```python
from build123d import *

# Parameters (mm, degrees)
SKETCH1_W                      = 70
SKETCH1_H                      = 310
BASE_FLANGE1_DEPTH             = 0.81
EDGE_FLANGE1_STRIP_W           = 4.7132
EDGE_FLANGE1_STRIP_H           = 0.81
EDGE_FLANGE1_STRIP_CUT_DEPTH   = 310
EDGE_FLANGE1_DEPTH             = 310
EDGE_FLANGE2_STRIP_W           = 4.7132
EDGE_FLANGE2_STRIP_H           = 0.81
EDGE_FLANGE2_STRIP_CUT_DEPTH   = 310
EDGE_FLANGE2_DEPTH             = 310
EDGE_FLANGE3_STRIP_W           = 4.7132
EDGE_FLANGE3_STRIP_H           = 0.81
EDGE_FLANGE3_STRIP_CUT_DEPTH   = 68.4534
EDGE_FLANGE3_STRIP_2_W         = 4.7132
EDGE_FLANGE3_STRIP_2_H         = 0.81
EDGE_FLANGE3_STRIP_CUT_2_DEPTH = 68.4534
EDGE_FLANGE3_DEPTH             = 68.4534
EDGE_FLANGE3_BEND_DEPTH        = 68.4534
CUT_EXTRUDE2_REACH             = 325.201
SKETCH18_R                     = 2.5
SKETCH18_R_2                   = 1.5
CUT_EXTRUDE1_REACH             = 325.201
SKETCH17_R                     = 17.5
SKETCH17_R_2                   = 2.5
SKETCH17_R_3                   = 6


# Sheet-metal steps are written as plain solids
with BuildPart() as part:
    # Sketch1 → Base-Flange1 (new body)
    with BuildSketch(Plane.XY):
        with Locations((35, 155)):
            Rectangle(SKETCH1_W, SKETCH1_H)
    extrude(amount=-BASE_FLANGE1_DEPTH)

    # Edge-Flange1 strip (across the edge) → Edge-Flange1 strip cut (cut)
    with BuildSketch(Plane(origin=(0, 0, -0.81), x_dir=(1, 0, 0), z_dir=(0, 1, 0))):
        with Locations((-0.81, -0.405)):
            Rectangle(EDGE_FLANGE1_STRIP_W, EDGE_FLANGE1_STRIP_H)
    extrude(amount=EDGE_FLANGE1_STRIP_CUT_DEPTH, mode=Mode.SUBTRACT)

    # Edge-Flange1 section (across the edge) → Edge-Flange1 (add)
    with BuildSketch(Plane(origin=(0, 0, -0.81), x_dir=(1, 0, 0), z_dir=(0, 1, 0))):
        with BuildLine():
            Line((0, 0.7366), (0, 58))
            Line((0, 58), (0.81, 58))
            Line((0.81, 58), (0.81, 0.7366))
            ThreePointArc((0.81, 0.7366), (1.025745145, 0.215745145), (1.5466, 0))
            Line((1.5466, 0), (1.5466, -0.81))
            ThreePointArc((1.5466, -0.81), (0.452988652, -0.357011348), (0, 0.7366))
        make_face()
    extrude(amount=EDGE_FLANGE1_DEPTH)

    # Edge-Flange2 strip (across the edge) → Edge-Flange2 strip cut (cut)
    with BuildSketch(Plane(origin=(0.81, 0, -58.81), x_dir=(0, 0, 1), z_dir=(0, 1, 0))):
        with Locations((-0.81, -0.405)):
            Rectangle(EDGE_FLANGE2_STRIP_W, EDGE_FLANGE2_STRIP_H)
    extrude(amount=EDGE_FLANGE2_STRIP_CUT_DEPTH, mode=Mode.SUBTRACT)

    # Edge-Flange2 section (across the edge) → Edge-Flange2 (add)
    with BuildSketch(Plane(origin=(0.81, 0, -58.81), x_dir=(0, 0, 1), z_dir=(0, 1, 0))):
        with BuildLine():
            Line((0, 0.7366), (0, 69.19))
            Line((0, 69.19), (0.81, 69.19))
            Line((0.81, 69.19), (0.81, 0.7366))
            ThreePointArc((0.81, 0.7366), (1.025745145, 0.215745145), (1.5466, 0))
            Line((1.5466, 0), (1.5466, -0.81))
            ThreePointArc((1.5466, -0.81), (0.452988652, -0.357011348), (0, 0.7366))
        make_face()
    extrude(amount=EDGE_FLANGE2_DEPTH)

    # Edge-Flange3 strip (across the edge) → Edge-Flange3 strip cut (cut)
    with BuildSketch(Plane(origin=(70, 0, -0.81), x_dir=(0, 1, 0), z_dir=(-1, 0, 0))):
        with Locations((-0.81, -0.405)):
            Rectangle(EDGE_FLANGE3_STRIP_W, EDGE_FLANGE3_STRIP_H)
    extrude(amount=EDGE_FLANGE3_STRIP_CUT_DEPTH, mode=Mode.SUBTRACT)

    # Edge-Flange3 strip 2 (across the edge) → Edge-Flange3 strip cut 2 (cut)
    with BuildSketch(Plane(origin=(1.5466, 0, -58), x_dir=(0, 1, 0), z_dir=(1, 0, 0))):
        with Locations((-0.81, -0.405)):
            Rectangle(EDGE_FLANGE3_STRIP_2_W, EDGE_FLANGE3_STRIP_2_H)
    extrude(amount=EDGE_FLANGE3_STRIP_CUT_2_DEPTH, mode=Mode.SUBTRACT)

    # Edge-Flange3 section (across the edge) → Edge-Flange3 (add)
    with BuildSketch(Plane(origin=(70, 0, -0.81), x_dir=(0, 1, 0), z_dir=(-1, 0, 0))):
        with BuildLine():
            Line((0, 0.7366), (0, 24.19))
            Line((0, 24.19), (0.81, 24.19))
            Line((0.81, 24.19), (0.81, 0.7366))
            ThreePointArc((0.81, 0.7366), (1.025745145, 0.215745145), (1.5466, 0))
            Line((1.5466, 0), (1.5466, -0.81))
            ThreePointArc((1.5466, -0.81), (0.452988652, -0.357011348), (0, 0.7366))
        make_face()
    extrude(amount=EDGE_FLANGE3_DEPTH)

    # Edge-Flange3 section 2 (across the edge) → Edge-Flange3 bend (add)
    with BuildSketch(Plane(origin=(1.5466, 0, -58), x_dir=(0, 1, 0), z_dir=(1, 0, 0))):
        with BuildLine():
            Line((0, 0.7366), (0, 24.19))
            Line((0, 24.19), (0.81, 24.19))
            Line((0.81, 24.19), (0.81, 0.7366))
            ThreePointArc((0.81, 0.7366), (1.025745145, 0.215745145), (1.5466, 0))
            Line((1.5466, 0), (1.5466, -0.81))
            ThreePointArc((1.5466, -0.81), (0.452988652, -0.357011348), (0, 0.7366))
        make_face()
    extrude(amount=EDGE_FLANGE3_BEND_DEPTH)

    # Sketch18 → Cut-Extrude2 (cut, up to next)
    with BuildSketch(Plane.XY.offset(-58.81), mode=Mode.PRIVATE) as cut_extrude2_sk1:
        with Locations(Location((37.83811715, 272.529876457, 0), (0, 0, 180))):
            Circle(SKETCH18_R)
    cut_extrude2_tool1 = extrude(cut_extrude2_sk1.sketch, amount=CUT_EXTRUDE2_REACH, mode=Mode.PRIVATE) & part.part
    # Sketch18 → Cut-Extrude2 (cut, up to next)
    with BuildSketch(Plane.XY.offset(-58.81), mode=Mode.PRIVATE) as cut_extrude2_sk2:
        with Locations(Location((50, 300, 0), (0, 0, 180))):
            Circle(SKETCH18_R)
    cut_extrude2_tool2 = extrude(cut_extrude2_sk2.sketch, amount=CUT_EXTRUDE2_REACH, mode=Mode.PRIVATE) & part.part
    # Sketch18 → Cut-Extrude2 (cut, up to next)
    with BuildSketch(Plane.XY.offset(-58.81), mode=Mode.PRIVATE) as cut_extrude2_sk3:
        with Locations(Location((37.721227194, 262.319243723, 0), (0, 0, 180))):
            Circle(SKETCH18_R_2)
    cut_extrude2_tool3 = extrude(cut_extrude2_sk3.sketch, amount=CUT_EXTRUDE2_REACH, mode=Mode.PRIVATE) & part.part
    # Sketch18 → Cut-Extrude2 (cut, up to next)
    with BuildSketch(Plane.XY.offset(-58.81), mode=Mode.PRIVATE) as cut_extrude2_sk4:
        with Locations(Location((37.83811715, 282.740509191, 0), (0, 0, 180))):
            Circle(SKETCH18_R_2)
    cut_extrude2_tool4 = extrude(cut_extrude2_sk4.sketch, amount=CUT_EXTRUDE2_REACH, mode=Mode.PRIVATE) & part.part
    # Sketch18 → Cut-Extrude2 (cut, up to next)
    with BuildSketch(Plane.XY.offset(-58.81), mode=Mode.PRIVATE) as cut_extrude2_sk5:
        with Locations(Location((15.605835414, 272.656798014, 0), (0, 0, 180))):
            Circle(SKETCH18_R_2)
    cut_extrude2_tool5 = extrude(cut_extrude2_sk5.sketch, amount=CUT_EXTRUDE2_REACH, mode=Mode.PRIVATE) & part.part
    add(cut_extrude2_tool1.solids().sort_by_distance((37.838117, 272.529876, -58.81))[0], mode=Mode.SUBTRACT)
    add(cut_extrude2_tool2.solids().sort_by_distance((50, 300, -58.81))[0], mode=Mode.SUBTRACT)
    add(cut_extrude2_tool3.solids().sort_by_distance((37.721227, 262.319244, -58.81))[0], mode=Mode.SUBTRACT)
    add(cut_extrude2_tool4.solids().sort_by_distance((37.838117, 282.740509, -58.81))[0], mode=Mode.SUBTRACT)
    add(cut_extrude2_tool5.solids().sort_by_distance((15.605835, 272.656798, -58.81))[0], mode=Mode.SUBTRACT)

    # Sketch17 → Cut-Extrude1 (cut, up to next)
    with BuildSketch(Plane(origin=(0, 0, 0), x_dir=(-1, 0, 0), z_dir=(0, 0, -1)), mode=Mode.PRIVATE) as cut_extrude1_sk1:
        with Locations((-29.120132649, 272.629176961)):
            Circle(SKETCH17_R)
    cut_extrude1_tool1 = extrude(cut_extrude1_sk1.sketch, amount=CUT_EXTRUDE1_REACH, mode=Mode.PRIVATE) & part.part
    # Sketch17 → Cut-Extrude1 (cut, up to next)
    with BuildSketch(Plane(origin=(0, 0, 0), x_dir=(-1, 0, 0), z_dir=(0, 0, -1)), mode=Mode.PRIVATE) as cut_extrude1_sk2:
        with Locations((-50, 300)):
            Circle(SKETCH17_R_2)
    cut_extrude1_tool2 = extrude(cut_extrude1_sk2.sketch, amount=CUT_EXTRUDE1_REACH, mode=Mode.PRIVATE) & part.part
    # Sketch17 → Cut-Extrude1 (cut, up to next)
    with BuildSketch(Plane(origin=(0, 0, 0), x_dir=(-1, 0, 0), z_dir=(0, 0, -1)), mode=Mode.PRIVATE) as cut_extrude1_sk3:
        with Locations((-35, 85)):
            Circle(SKETCH17_R_3)
    cut_extrude1_tool3 = extrude(cut_extrude1_sk3.sketch, amount=CUT_EXTRUDE1_REACH, mode=Mode.PRIVATE) & part.part
    # Sketch17 → Cut-Extrude1 (cut, up to next)
    with BuildSketch(Plane(origin=(0, 0, 0), x_dir=(-1, 0, 0), z_dir=(0, 0, -1)), mode=Mode.PRIVATE) as cut_extrude1_sk4:
        with BuildLine():
            Line((-43.15, 43.5), (-39.873397172, 43.5))
            ThreePointArc((-39.873397172, 43.5), (-35, 46), (-30.126602828, 43.5))
            Line((-30.126602828, 43.5), (-26.85, 43.5))
            ThreePointArc((-26.85, 43.5), (-23.35, 40), (-26.85, 36.5))
            Line((-26.85, 36.5), (-30.126602828, 36.5))
            ThreePointArc((-30.126602828, 36.5), (-35, 34), (-39.873397172, 36.5))
            Line((-39.873397172, 36.5), (-43.15, 36.5))
            ThreePointArc((-43.15, 36.5), (-46.65, 40), (-43.15, 43.5))
        make_face()
    cut_extrude1_tool4 = extrude(cut_extrude1_sk4.sketch, amount=CUT_EXTRUDE1_REACH, mode=Mode.PRIVATE) & part.part
    add(cut_extrude1_tool1.solids().sort_by_distance((29.120133, 272.629177, 0))[0], mode=Mode.SUBTRACT)
    add(cut_extrude1_tool2.solids().sort_by_distance((50, 300, 0))[0], mode=Mode.SUBTRACT)
    add(cut_extrude1_tool3.solids().sort_by_distance((35, 85, 0))[0], mode=Mode.SUBTRACT)
    add(cut_extrude1_tool4.solids().sort_by_distance((35, 40, 0))[0], mode=Mode.SUBTRACT)


solid = part.part
```
Model file for the job. Use its own axes, mm. A direction names the side the tool comes from. Coordinates: 2 decimals unless noted, no trailing zeros. Write each loop counter-clockwise with the first axis right and the second up, starting at its lowest first coordinate (ties: lowest second). Pieces come first, ordered by that corner, then holes. Notation, with made-up numbers: (50, 23) - (67, 23) arc R25 cw to (67, 52) - close; hole circle Ø1 at (10.5, 77.5). An arc over 180 degrees is marked (long way). Use a Markdown table: item, result. Add a question column.
Item 1: Band-saw the part on D-D, the plane y = 85. Write the cut outline in (x, z).
Item 2: 3-axis set-ups, long thin cutter, end or side, ignore diameter. For faces 1 (the face through (39.42, 89.06, -0.4)), 2 (the face through (35, 158, -0.81)), 3 (the face through (35, 154, -58.81)): which of +Z, -Z, +X, -X, +Y, -Y reach the whole face in a straight line?
Item 3: Two-plate mould, pull along Z, no slides. Class faces 4 (the face through (35, 158, 0)), 5 (the face through (36, 154, -58)), 6 (the face through (0, 153, -29)): pulls with the +Z half, pulls with the -Z half, needs draft (parallel to the pull), parting line crosses it, or undercut.
Item 4: Band-saw the part on A-A, the plane y = 40. Write the cut outline in (x, z), and give its area (3 significant figures).
Item 5: Band-saw the part on B-B, the plane z = -15. Write the cut outline in (x, y), and give its area (3 significant figures).
Item 6: Band-saw the part on C-C, the plane y = 207. Write the cut outline in (x, z), and give its area (3 significant figures).
Item 7: Drill centre lines: line 1 along Z through (x, y) = (9, 85); line 2 along Y through (x, z) = (8.5, -16). Where is each one in solid material? Low to high.
Item 8: Drop flat-ended pins along their axis: pin 1 (12 mm diameter, centred on x = 8.5, z = -47.5, fed in from +Y); pin 2 (4 mm diameter, centred on x = 26, y = 141.5, fed in from +Z); pin 3 (1.5 mm diameter, centred on y = 236.5, z = -40.5, fed in from +X); pin 4 (6 mm diameter, centred on x = 37.84, y = 272.53, fed in from +Z). Give the stop position or say it passes through.
A:
| question | item | result |
|---|---|---|
| 1 | outline | (0, -57.26) arc R1.55 ccw to (1.55, -58.81) - (70, -58.81) - (70, -58) - (1.55, -58) arc R0.74 cw to (0.81, -57.26) - (0.81, -1.55) arc R0.74 cw to (1.55, -0.81) - (29, -0.81) - (29, 0) - (1.55, 0) arc R1.55 ccw to (0, -1.55) - close; (41, -0.81) - (70, -0.81) - (70, 0) - (41, 0) - close |
| 2 | face 1 | +Z |
| 2 | face 2 | +X, +Y |
| 2 | face 3 | -Z, +X, -X, +Y, -Y |
| 3 | face 4 | pulls with the +Z half |
| 3 | face 5 | undercut |
| 3 | face 6 | needs draft |
| 4 | outline | (0, -57.26) arc R1.55 ccw to (1.55, -58.81) - (70, -58.81) - (70, -58) - (1.55, -58) arc R0.74 cw to (0.81, -57.26) - (0.81, -1.55) arc R0.74 cw to (1.55, -0.81) - (23.35, -0.81) - (23.35, 0) - (1.55, 0) arc R1.55 ccw to (0, -1.55) - close; (46.65, -0.81) - (70, -0.81) - (70, 0) - (46.65, 0) - close |
| 4 | area | 140 mm² |
| 5 | outline | (0, 0) - (0.81, 0) - (0.81, 310) - (0, 310) - close; (1.55, 0) - (70, 0) - (70, 0.81) - (1.55, 0.81) - close |
| 5 | area | 307 mm² |
| 6 | outline | (0, -57.26) arc R1.55 ccw to (1.55, -58.81) - (70, -58.81) - (70, -58) - (1.55, -58) arc R0.74 cw to (0.81, -57.26) - (0.81, -1.55) arc R0.74 cw to (1.55, -0.81) - (70, -0.81) - (70, 0) - (1.55, 0) arc R1.55 ccw to (0, -1.55) - close |
| 6 | area | 159 mm² |
| 7 | line 1 | z = -58.81 to -58, -0.81 to 0 |
| 7 | line 2 | y = 0 to 0.81 |
| 8 | pin 1 | stops at y = 0.81 |
| 8 | pin 2 | stops at z = 0 |
| 8 | pin 3 | stops at x = 0.81 |
| 8 | pin 4 | stops at z = -58 |
